from build123d import *

# Parameters (mm, degrees)
CHAFL_N2_SIZE         = 0.3
CHAFL_N2_SIZE2        = 0.212132034
CHAFL_N3_SIZE         = 0.3
CORTAR_EXTRUIR2_DEPTH = 1


with BuildPart() as part:
    # Croquis1 → Revolución1 (revolve)
    with BuildSketch(Plane.XY, mode=Mode.PRIVATE) as revoluci_n1_sk:
        Polygon((0, 0), (3.2, 0), (1.5, -1.7), (1.5, -10), (0, -10), align=None)
    revolve(revoluci_n1_sk.sketch.rotate(Axis((0, 0, 0), (0, -1, 0)), 90), axis=Axis((0, 0, 0), (0, -1, 0)))

    # Chaflán2
    chafl_n2_edges = [part.edges().sort_by_distance(p)[0] for p in [
        (0, 0, -3.2),
    ]]
    chafl_n2_side = [part.faces().sort_by_distance(p)[0] for p in [
        (0, -0.85, -2.35),
    ]]
    chamfer(chafl_n2_edges, length=CHAFL_N2_SIZE, length2=CHAFL_N2_SIZE2, reference=chafl_n2_side[0])

    # Chaflán3
    chafl_n3_edges = [part.edges().sort_by_distance(p)[0] for p in [
        (0, -10, -1.5),
    ]]
    chamfer(chafl_n3_edges, length=CHAFL_N3_SIZE)

    # Croquis3 → Cortar-Extruir2 (cut)
    with BuildSketch(Plane(origin=(0, 0, 0), x_dir=(1, 0, 0), z_dir=(0, 1, 0))):
        Polygon((-0.721687836, 1.25), (-1.443375673, 0), (-0.721687836, -1.25), (0.721687836, -1.25), (1.443375673, 0), (0.721687836, 1.25), align=None)
    extrude(amount=-CORTAR_EXTRUIR2_DEPTH, mode=Mode.SUBTRACT)


solid = part.part
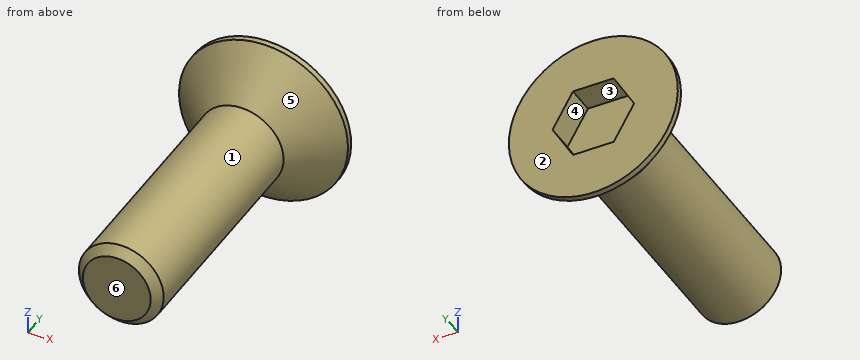
Read the model definition and answer for the solid it produces. Units are mm, in the model's axes. Face numbers are marked on the shaded views. A direction names the side the tool comes from. Round coordinates to 2 decimals unless told otherwise and drop trailing zeros. Write each loop counter-clockwise with the first axis right and the second up, starting at its lowest first coordinate (ties: lowest second). Pieces come first, ordered by that corner, then holes.
1. Which of the six approach directions +Z, -Z, +X, -X, +Y, -Y give full straight-line access (tool end or side, diameter ignored) to the marked faces 1, 2 and 3?
2. Determine the mould class of the marked faces 4, 5 and 6 for opening direction Z: pulls with the +Z half, pulls with the -Z half, needs draft (parallel to the pull), parting line crosses it, or undercut.
3. Given pin 1 Ø1 at (x, y) = (-0.5, -6) entering from -Z; pin 2 Ø2 at (x, z) = (-2, 1) entering from -Y; pin 3 Ø1.2 at (x, z) = (0.5, 0) entering from +Y, each flat-ended and moving along its own axis, determine where each tip first touches the part or whether it passes through.
4. Straight lines are drawn through the part: L1, parallel to X at y = -3.75, z = -0.4; L2, parallel to X at y = -3.25, z = -0.1; L3, parallel to Y at x = 0.7, z = -0.1. For each, find the intervals that lie inside material, in ascending order.
5. The part is cut by section A-A, the plane y = -3.5. Determine the outline of the cut face in (x, z).
Values:
1. face 1: -Y
1. face 2: +Z, -Z, +X, -X, +Y
1. face 3: +Y
2. face 4: undercut
2. face 5: parting line crosses it
2. face 6: needs draft
3. pin 1: stops at z = -1.5
3. pin 2: stops at y = -9.96
3. pin 3: stops at y = -1
4. L1: x = -1.45 to 1.45
4. L2: x = -1.5 to 1.5
4. L3: y = -10 to -1
5. outline: circle Ø3 at (0, 0)
